Source: CAD feature listing. Evaluate the final solid. Frame: model axes, mm. A direction names the side the tool comes from. Give positions to 0.01 mm unless a question says otherwise; leave off trailing zeros. Loops run counter-clockwise (first coordinate to the right, second up) from the corner with the lowest first, then second, coordinate; pieces in that order, holes last.
from build123d import *

# Parameters (mm, degrees)
BOSS_EXTRUDE1_DEPTH = 2


with BuildPart() as part:
    # Sketch1 → Boss-Extrude1 (new body)
    with BuildSketch(Plane.XY):
        with BuildLine():
            Line((-6, 0), (-6, -27))
            ThreePointArc((-6, -27), (-5.121320344, -29.121320344), (-3, -30))
            Line((-3, -30), (3, -30))
            ThreePointArc((3, -30), (5.121320344, -29.121320344), (6, -27))
            Line((6, -27), (6, 0))
            ThreePointArc((6, 0), (0, 6), (-6, 0))
        make_face()
        with BuildLine():
            Line((-2.236067977, 2), (2.236067977, 2))
            ThreePointArc((2.236067977, 2), (0, -3), (-2.236067977, 2))
        make_face(mode=Mode.SUBTRACT)
    extrude(amount=BOSS_EXTRUDE1_DEPTH)


solid = part.part
1) Cut plane B-B (z = 1). Return loops of the section in (x, y), and give its area (3 significant figures).
Checks:
outline: (-6, -27) arc R3 ccw to (-3, -30) - (3, -30) arc R3 ccw to (6, -27) - (6, 0) arc R6 ccw to (-6, 0) - close; hole (-2.24, 2) arc R3 ccw (long way) to (2.24, 2) - close
area: 388 mm2
2) Pull-direction query (Y, two-part tool) for faces 3 (the cylindrical face through (0, -3, 1)), 4 (the cylindrical face through (-5.14, -29.1, 0.99)), 5 (the flat face through (0, -12, 2)); classes: released by +Y, released by -Y, zero draft, split by the parting line, or undercut.
Checks:
face 3: undercut
face 4: released by -Y
face 5: zero draft
3) Ray query, probe 1 along Y at (x, z) = (0, 0.8); probe 2 along X at (y, z) = (0, 1.35); probe 3 along Y at (x, z) = (1.75, 0.75). Return the intervals inside material, ascending.
Checks:
probe 1: y = -30 to -3, 2 to 6
probe 2: x = -6 to -3, 3 to 6
probe 3: y = -30 to -2.44, 2 to 5.74
4) Reachability of faces 1 (the flat face through (0, -12, 0)), 2 (the flat face through (0, 2, 1)) from +Z, -Z, +X, -X, +Y, -Y: full face, straight path, thin tool, end or side. Return the list, or none.
Checks:
face 1: -Z, +X, -X, +Y, -Y
face 2: +Z, -Z
5) Cut plane D-D (y = 3.5). Return loops of the section in (x, z).
Checks:
outline: (-4.87, 0) - (4.87, 0) - (4.87, 2) - (-4.87, 2) - close
6) Cut plane C-C (y = -1). Return loops of the section in (x, z), and give its area (3 significant figures).
Checks:
outline: (-6, 0) - (-2.83, 0) - (-2.83, 2) - (-6, 2) - close; (2.83, 0) - (6, 0) - (6, 2) - (2.83, 2) - close
area: 12.7 mm2
7) Cut plane A-A (x = 0). Return loops of the section in (y, z), and give its area (3 significant figures).
Checks:
outline: (-30, 0) - (-3, 0) - (-3, 2) - (-30, 2) - close; (2, 0) - (6, 0) - (6, 2) - (2, 2) - close
area: 62.0 mm2
